Input: part model. Units: mm. Frame: model coordinates. Face numbers are marked on the shaded views. A direction names the side the tool comes from. Coordinates: 2 decimals unless noted, no trailing zeros. Loops run counter-clockwise (first coordinate to the right, second up) from the corner with the lowest first, then second, coordinate; pieces in that order, holes last. Notation, with made-up numbers: (14.5, -18.75) -> (37.5, -18.75) arc R19 cw to (37.5, -11.75) -> close; hole circle Ø2 at (51.5, 83). An arc over 180 degrees is marked (long way). Put each result on its own line as item: value. Start each with the question number.
1) Material intervals for L1, parallel to X at y = 37, z = -4.5; L2, parallel to X at y = -30.5, z = -1.75; L3, parallel to Z at x = 4.25, y = -38.5, sorted ascending.
2) Cut plane B-B (x = -0.1). Return the cut outline in (y, z).
3) Set-up query: the marked faces 1 and 2. Return all of +Z, -Z, +X, -X, +Y, -Y with unobstructed straight access to the full face (end or side cutting, diameter ignored); none if empty.
4) Cut plane C-C (y = -6). Return the cut outline in (x, z), plus the area to 3 significant figures.
5) Contact query for flat-ended pins moving along their axis: P1, Ø4, axis at x = 2, y = -15, coming from the +Z side; P2, Ø3, axis at y = -25, z = 4.5, coming from the +X side; P3, Ø1, axis at x = -4.5, y = -11, coming from the -Z side. Output: stop coordinate, or through.
6) Cut plane A-A (z = 0). Return the cut outline in (x, y).
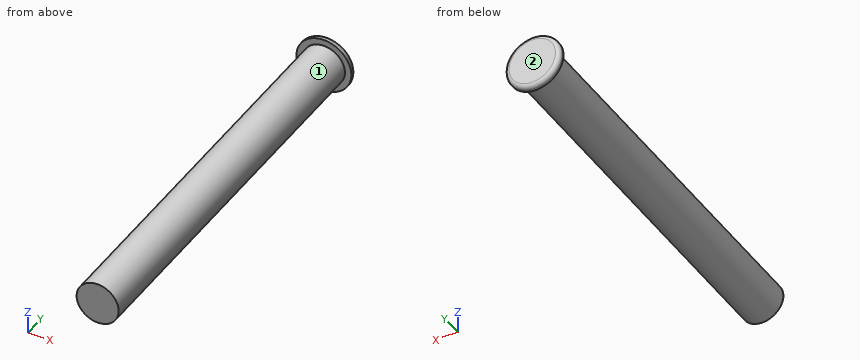
from build123d import *

# Parameters (mm, degrees)
SKETCH011_R       = 4.9
PAD002_DEPTH      = 44.95
CYLINDER003_R     = 6.4
CYLINDER003_DEPTH = 1.5
FILLET_R          = 1


with BuildPart() as part:
    # Sketch011 → Pad002 (new body, symmetric)
    with BuildSketch(Plane.XZ):
        with Locations((-0.1, 0)):
            Circle(SKETCH011_R)
    extrude(amount=PAD002_DEPTH, both=True)

    # Cylinder003 → Cylinder003 (join)
    with BuildSketch(Plane(origin=(-0.1, 44.95, 0), x_dir=(1, 0, 0), z_dir=(0, 1, 0))):
        Circle(CYLINDER003_R)
    extrude(amount=CYLINDER003_DEPTH)

    # Fillet
    fillet_edges = [part.edges().sort_by_distance(p)[0] for p in [
        (-6.5, 46.45, 0),
    ]]
    fillet(fillet_edges, radius=FILLET_R)


solid = part.part
Results found:
1. L1: x = -2.04 to 1.84
1. L2: x = -4.68 to 4.48
1. L3: z = -2.26 to 2.26
2. outline: (-44.95, -4.9) -> (44.95, -4.9) -> (44.95, -6.4) -> (45.45, -6.4) arc R1 ccw to (46.45, -5.4) -> (46.45, 5.4) arc R1 ccw to (45.45, 6.4) -> (44.95, 6.4) -> (44.95, 4.9) -> (-44.95, 4.9) -> close
3. face 1: -Y
3. face 2: +Z, -Z, +X, -X, +Y
4. outline: circle Ø9.8 at (-0.1, 0)
4. area: 75.4 mm2
5. P1: stops at z = 4.9
5. P2: stops at x = 3.77
5. P3: stops at z = -2.97
6. outline: (-6.5, 44.95) -> (-5, 44.95) -> (-5, -44.95) -> (4.8, -44.95) -> (4.8, 44.95) -> (6.3, 44.95) -> (6.3, 45.45) arc R1 ccw to (5.3, 46.45) -> (-5.5, 46.45) arc R1 ccw to (-6.5, 45.45) -> close
